Job drawing, mm, ordinate dimensions from the low corner. One solid piece. Give positions to 0.01 mm unless a question says otherwise; leave off trailing zeros. Write each loop counter-clockwise with the first axis right and the second up, starting at its lowest first coordinate (ties: lowest second). Pieces come first, ordered by that corner, then holes. Notation, with made-up numbers: (-12.5, 56) -> (34.5, 56) arc R21 cw to (34.5, 75) -> close; hole circle Ø3 at (69.25, -13). An arc over 180 degrees is marked (long way). Put each result on its own line as item: value. Start each with the question number.
Item 1: Slice it at B-B, the plane x = 47. List the corners of the cut face in (y, z).
Item 2: Slice it at C-C, the plane z = 90.5. List the corners of the cut face in (x, y), plus the area to 3 significant figures.
Item 3: Slice it at A-A, the plane z = 59. List the corners of the cut face in (x, y).
Item 4: Slice it at D-D, the plane y = 4.4. Give the number of separate pieces and of enclosed holes in the cut face, plus the area to 3 significant figures.
Item 5: Drill centre lines: line 1 along X through (y, z) = (3.1, 59); line 2 along Z through (x, y) = (56, 4.25); line 3 along Z through (x, y) = (18, 0.3). Where is each one in solid material? Low to high.
Item 6: Flat gauge pins, fed straight in: pin 1 Ø1.8 at (y, z) = (4, 2) entering from +X; pin 2 Ø3 at (x, y) = (14, 2.5) entering from +Z; pin 3 Ø18 at (x, z) = (20, 26) entering from +Y; pin 4 Ø1.8 at (x, y) = (6.5, 2.5) entering from -Z. Where does each tip first touch, or does it go through?
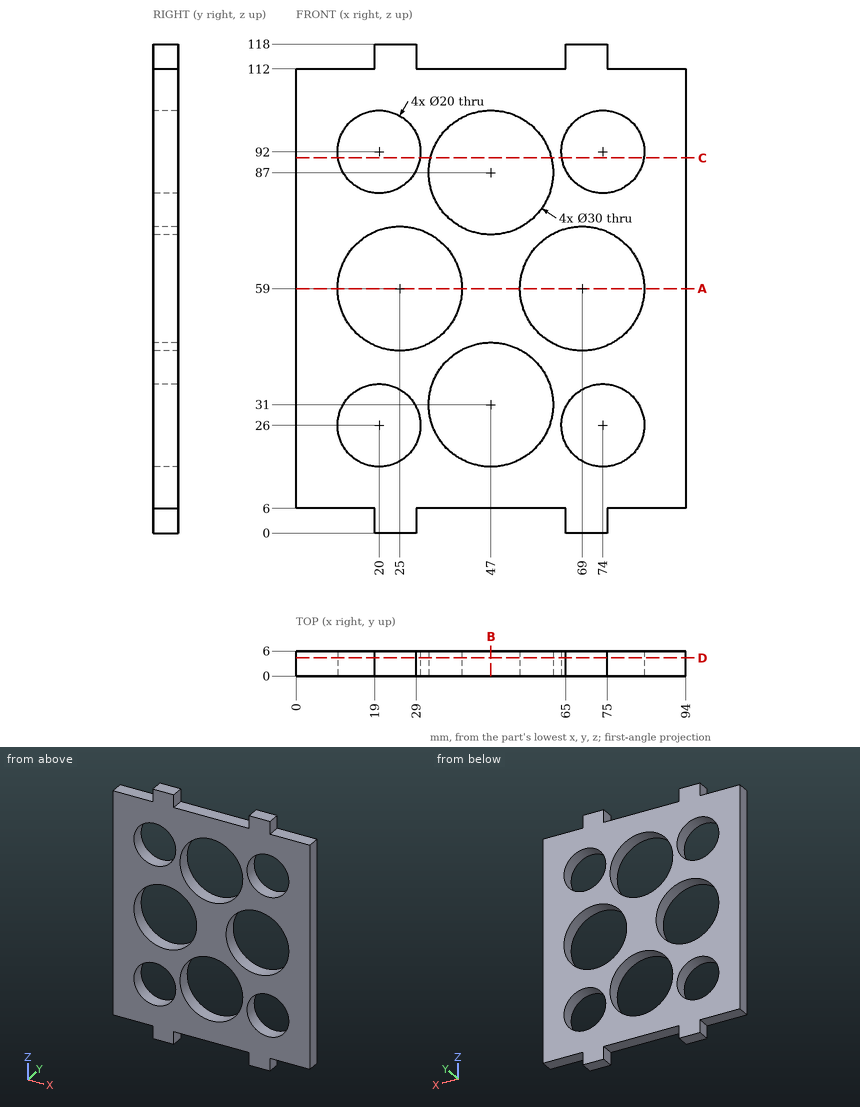
Values follow:
1. outline: (0, 6) -> (6, 6) -> (6, 16) -> (0, 16) -> close; (0, 46) -> (6, 46) -> (6, 72) -> (0, 72) -> close; (0, 102) -> (6, 102) -> (6, 112) -> (0, 112) -> close
2. outline: (0, 0) -> (10.11, 0) -> (10.11, 6) -> (0, 6) -> close; (29.89, 0) -> (32.41, 0) -> (32.41, 6) -> (29.89, 6) -> close; (61.59, 0) -> (64.11, 0) -> (64.11, 6) -> (61.59, 6) -> close; (83.89, 0) -> (94, 0) -> (94, 6) -> (83.89, 6) -> close
2. area: 152 mm2
3. outline: (0, 0) -> (10, 0) -> (10, 6) -> (0, 6) -> close; (40, 0) -> (54, 0) -> (54, 6) -> (40, 6) -> close; (84, 0) -> (94, 0) -> (94, 6) -> (84, 6) -> close
4. separate pieces: 1
4. enclosed holes: 8
4. area: 6,120 mm2
5. line 1: 0 to 10, 40 to 54, 84 to 94
5. line 2: 6 to 19, 43 to 51.52, 66.48 to 75, 99 to 112
5. line 3: 6 to 16.2, 35.8 to 45.73, 72.27 to 82.2, 101.8 to 112
6. pin 1: x = 75
6. pin 2: z = 112
6. pin 3: through
6. pin 4: z = 6
